Check sheet for the modelled part. Datum: model origin and axes. Units: mm. A direction names the side the tool comes from. Round coordinates to 2 decimals unless told otherwise and drop trailing zeros. Order: outer loops, then holes, each group sorted by start corner. A loop starts at its lowest first (then second) coordinate and runs counter-clockwise, first axis right, second up. Notation, with made-up numbers: (17, 66) -> (61, 66) arc R14 cw to (61, 87) -> close; hole circle Ø5 at (68, 71.25). An arc over 180 degrees is marked (long way). Answer in a Markdown table with one row per item. Add a question column.
1. Draft check along Y on faces 1 (the flat face through (-46, 90, 1)), 2 (the flat face through (-30, 30, 1)), 3 (the flat face through (-90, 44, 1)), 4 (the flat face through (-60, 30, 1)). Enter one of: +Y half, -Y half, draft (parallel to the pull), parting line (faces both ways), or undercut.
2. Sectioned sample at C-C, the plane y = 17.5. Record the boundary of the cut face in (x, z), then the cut area to 3 significant figures.
3. Access from +Z, -Z, +X, -X, +Y, -Y to the whole of each face (thin tool, end or side, straight path). Record for faces 5 (the flat face through (-45, 15, 1)), 6 (the flat face through (0, 44, 1)).
4. Material ranges on L1, parallel to X at y = 18.5, z = 1.05; L2, parallel to Y at x = -47.5, z = 2.4, recorded low to high. Write a range as from..to.
5. Depth check by flat-ended pin: P1, Ø2, axis at x = -58, y = 20.5, coming from the +Z side. Enter the tip coordinate at first touch or a pass-through.
6. Sectioned sample at B-B, the plane z = 1.1. Record the boundary of the cut face in (x, y), then the cut area to 3 significant figures.
7. Sectioned sample at A-A, the plane x = -40.5. Record the boundary of the cut face in (y, z).
```python
from build123d import *

# Parameters (mm, degrees)
SKETCH_W     = 90
SKETCH_H     = 90
PAD_DEPTH    = 3
SKETCH001_W  = 30
SKETCH001_H  = 30
POCKET_DEPTH = 3


with BuildPart() as part:
    # Sketch → Pad (new body)
    with BuildSketch(Plane.XY):
        with Locations((-45, 45)):
            Rectangle(SKETCH_W, SKETCH_H)
    extrude(amount=PAD_DEPTH)

    # Sketch001 → Pocket (cut)
    with BuildSketch(Plane.XY):
        with Locations((-45, 30)):
            Rectangle(SKETCH001_W, SKETCH001_H)
    extrude(amount=POCKET_DEPTH, mode=Mode.SUBTRACT)


solid = part.part
```
Answer key:
| question | item | result |
|---|---|---|
| 1 | face 1 | +Y half |
| 1 | face 2 | undercut |
| 1 | face 3 | draft |
| 1 | face 4 | undercut |
| 2 | outline | (-90, 0) -> (-60, 0) -> (-60, 3) -> (-90, 3) -> close; (-30, 0) -> (0, 0) -> (0, 3) -> (-30, 3) -> close |
| 2 | area | 180 mm² |
| 3 | face 5 | +Z, -Z |
| 3 | face 6 | +Z, -Z, +X, +Y, -Y |
| 4 | L1 | x = -90..-60, -30..0 |
| 4 | L2 | y = 0..15, 45..90 |
| 5 | P1 | passes through |
| 6 | outline | (-90, 0) -> (0, 0) -> (0, 90) -> (-90, 90) -> close; hole (-60, 15) -> (-30, 15) -> (-30, 45) -> (-60, 45) -> close |
| 6 | area | 7,200 mm² |
| 7 | outline | (0, 0) -> (15, 0) -> (15, 3) -> (0, 3) -> close; (45, 0) -> (90, 0) -> (90, 3) -> (45, 3) -> close |
